Autodesk Inventor part; units mm, degrees
ref_plane "YZ Plane" through (0, 0, 0) normal (1, 0, 0) x (0, 1, 0)
ref_plane "XZ Plane" through (0, 0, 0) normal (0, 1, 0) x (-1, 0, 0)
ref_plane "XY Plane" through (0, 0, 0) normal (0, 0, 1) x (1, 0, 0)
sketch "Sketch1" plane through (0, 0, 0) normal (0, 0, 1) x (1, 0, 0)
  circle A0 centre (3.2816, -5.4552) radius 1.5
  line L0 (4.45, -12.0667) -> (7.65, -10.2192)
  line L1 (7.65, -10.2192) -> (10.85, -12.0667)
  line L2 (10.85, -12.0667) -> (10.85, -15.7617)
  line L3 (10.85, -15.7617) -> (7.65, -17.6093)
  line L4 (7.65, -17.6093) -> (4.45, -15.7617)
  line L5 (4.45, -15.7617) -> (4.45, -12.0667)
  circle A1 centre (3.2816, -22.3733) radius 1.5
  line L6 (15.3, -27.8284) -> (15.3, 0)
  line L7 (0, 0) -> (15.3, 0)
  line L8 (0, -27.8284) -> (0, 0)
  line L9 (0, -27.8284) -> (15.3, -27.8284)
  line L10 (28.3, 5.8858) -> (15.3, 5.8858)
  line L11 (15.3, 5.8858) -> (15.3, -34.1142)
  line L12 (28.3, -34.1142) -> (15.3, -34.1142)
  line L13 (28.3, 5.8858) -> (28.3, -34.1142)
  line L14 (38.8108, -39.1142) -> (38.8108, 10.8858)
  line L15 (38.8108, 10.8858) -> (15.3, 10.8858)
  line L16 (15.3, -2.6142) -> (15.3, 10.8858)
  line L17 (15.3, -2.6142) -> (38.3, -2.6142)
  line L18 (38.3, -12.6142) -> (38.3, -2.6142)
  line L19 (38.3, -12.6142) -> (7.65, -12.6142)
  arc A2 (7.65, -15.6142) -> (7.65, -12.6142) centre (7.65, -14.1142) ccw
  line L20 (7.65, -15.6142) -> (38.3, -15.6142)
  line L21 (38.3, -25.6142) -> (38.3, -15.6142)
  line L22 (38.3, -25.6142) -> (15.3, -25.6142)
  line L23 (15.3, -39.1142) -> (15.3, -25.6142)
  line L24 (38.8108, -39.1142) -> (15.3, -39.1142)
  line L25 (-7.04, -39.1142) -> (14.96, -39.1142)
  line L26 (-7.04, -39.1142) -> (38.8108, -39.1142)
  line L27 (38.8108, -39.1142) -> (38.8108, 10.8858)
  line L28 (38.8108, 10.8858) -> (-7.04, 10.8858)
  line L29 (-7.04, 10.8858) -> (-7.04, -39.1142)
  line L30 (-5.04, -27.8284) -> (13.16, -27.8284)
  line L31 (13.16, 0) -> (-5.04, 0)
  line L32 (-3.04, -35.1142) -> (34.8108, -35.1142)
  line L33 (34.8108, -35.1142) -> (34.8108, 6.8858)
  line L34 (34.8108, 6.8858) -> (-3.04, 6.8858)
  line L35 (-3.04, 6.8858) -> (-3.04, -35.1142)
  line L36 (34.8108, -35.1142) -> (15.3, -35.1142)
  line L37 (15.3, -35.1142) -> (15.3, -39.1142)
  line L38 (15.3, -39.1142) -> (34.8108, -39.1142)
  line L39 (34.8108, -39.1142) -> (34.8108, -35.1142)
  line L40 (15.3, 6.8858) -> (34.8108, 6.8858)
  line L41 (34.8108, 6.8858) -> (34.8108, 10.8858)
  line L42 (34.8108, 10.8858) -> (15.3, 10.8858)
  line L43 (15.3, 10.8858) -> (15.3, 6.8858)
  point P0 (-3.04, 0)
  point P1 (-3.04, -27.8284)
  dimension "d0" = 4
extrude "Extrusion1" add sketch "Sketch1" along normal blind 2 contours L5 L4 L3 L2 L20 L6 L9 L8 L7 L19 L1 L0 | L0 L1 L2 L19 A2 L20 L3 L4 L5 | L19 L6 L20 L2 | L2 L20 A2 L19 | L19 L13 L20 L6 | L6 L17 L13 L19 | L20 L13 L22 L6 | L6 L11 L10 L13 L17 | L19 L33 L20 L13 | L13 L17 L33 L19 | L22 L13 L12 L11 L6 | L20 L33 L22 L13 | L13 L10 L16 L34 L33 L17 | L33 L17 L18 L19 | L19 L18 L17 L33 L41 L15 L14 L24 L39 L22 L21 L20 | L22 L33 L32 L23 L12 L13 | L20 L21 L22 L33 | L8 L30 L35 L31 | L16 L15 L41 L34 | L32 L39 L24 L23
sketch "Sketch2" plane through (0, 0, 2) normal (0, 0, 1) x (1, 0, 0)
  line L0 (15.3, 0) -> (-3.04, 0)
  line L1 (-3.04, 0) -> (-3.04, -27.8284)
  line L2 (-3.04, -27.8284) -> (15.3, -27.8284)
  line L3 (15.3, -27.8284) -> (15.3, -39.1142)
  line L4 (15.3, -39.1142) -> (38.8108, -39.1142)
  line L5 (38.8108, -39.1142) -> (38.8108, 10.8858)
  line L6 (38.8108, 10.8858) -> (15.3, 10.8858)
  line L7 (15.3, 10.8858) -> (15.3, 0)
  circle A0 centre (3.2816, -22.3733) radius 1.5
  circle A1 centre (3.2816, -5.4552) radius 1.5
  line L8 (15.3, -39.1142) -> (38.8108, -39.1142)
  line L9 (38.8108, 10.8858) -> (34.8108, 10.8858)
  line L10 (34.8108, 10.8858) -> (34.8108, -39.1142)
  line L11 (34.8108, -39.1142) -> (38.8108, -39.1142)
  line L12 (38.8108, -39.1142) -> (38.8108, 10.8858)
  point P0 (0, 0)
  dimension "d3" = 4
extrude "Extrusion2" cut sketch "Sketch2" against normal blind 2 contours L6 L5 L4 L10
sketch "Sketch3" plane through (0, 0, 2) normal (0, 0, 1) x (1, 0, 0)
  point P0 (0, 0)
sketch "Sketch4" plane through (0, 0, 2) normal (0, 0, 1) x (1, 0, 0)
  circle A0 centre (16.8, -32.0784) radius 0.75
  circle A1 centre (16.8, 4.25) radius 0.75
  point P0 (0, 0)
extrude "Extrusion3" cut sketch "Sketch4" against normal through all
sketch "Sketch5" plane through (0, 0, 2) normal (0, 0, 1) x (1, 0, 0)
  circle A0 centre (16.8, 4.25) radius 0.75
  circle A1 centre (16.8, -32.0784) radius 0.75
  line L0 (34.8108, -39.1142) -> (34.8108, 10.8858)
  line L1 (34.8108, 10.8858) -> (15.3, 10.8858)
  line L2 (15.3, 10.8858) -> (15.3, 0)
  line L3 (15.3, 0) -> (-3.04, 0)
  line L4 (-3.04, 0) -> (-3.04, -27.8284)
  line L5 (-3.04, -27.8284) -> (15.3, -27.8284)
  line L6 (15.3, -27.8284) -> (15.3, -39.1142)
  line L7 (15.3, -39.1142) -> (34.8108, -39.1142)
  circle A2 centre (3.2816, -22.3733) radius 1.5
  circle A3 centre (3.2816, -5.4552) radius 1.5
  line L8 (22.1108, -36.7142) -> (32.8108, -36.7142)
  line L9 (22.1108, -36.7142) -> (22.1108, -35.1142)
  line L10 (32.8108, -35.1142) -> (22.1108, -35.1142)
  line L11 (32.8108, -36.7142) -> (32.8108, -35.1142)
  line L12 (32.4108, -28.3142) -> (32.4108, -17.6142)
  line L13 (32.4108, -28.3142) -> (30.8108, -28.3142)
  line L14 (30.8108, -17.6142) -> (30.8108, -28.3142)
  line L15 (32.4108, -17.6142) -> (30.8108, -17.6142)
  line L16 (32.4108, -6.3142) -> (32.4108, 4.3858)
  line L17 (32.4108, -6.3142) -> (30.8108, -6.3142)
  line L18 (30.8108, 4.3858) -> (30.8108, -6.3142)
  line L19 (32.4108, 4.3858) -> (30.8108, 4.3858)
  line L20 (32.8108, 8.4858) -> (22.1108, 8.4858)
  line L21 (32.8108, 8.4858) -> (32.8108, 6.8858)
  line L22 (22.1108, 6.8858) -> (32.8108, 6.8858)
  line L23 (22.1108, 8.4858) -> (22.1108, 6.8858)
  point P0 (0, 0)
extrude "Extrusion4" cut sketch "Sketch5" against normal through all contours L9 L10 L11 L8 | L13 L14 L15 L12 | L17 L18 L19 L16 | L21 L22 L23 L20
sketch "Sketch6" plane through (0, 0, 2) normal (0, 0, 1) x (1, 0, 0)
  line L0 (30.8108, -28.3142) -> (30.8108, -17.6142)
  line L1 (30.8108, -17.6142) -> (32.4108, -17.6142)
  line L2 (32.4108, -17.6142) -> (32.4108, -28.3142)
  line L3 (32.4108, -28.3142) -> (30.8108, -28.3142)
  line L4 (30.8108, -6.3142) -> (30.8108, 4.3858)
  line L5 (30.8108, 4.3858) -> (32.4108, 4.3858)
  line L6 (32.4108, 4.3858) -> (32.4108, -6.3142)
  line L7 (32.4108, -6.3142) -> (30.8108, -6.3142)
  line L8 (22.1108, -35.1142) -> (32.8108, -35.1142)
  line L9 (32.8108, -35.1142) -> (32.8108, -36.7142)
  line L10 (32.8108, -36.7142) -> (22.1108, -36.7142)
  line L11 (22.1108, -36.7142) -> (22.1108, -35.1142)
  line L12 (32.8108, 6.8858) -> (22.1108, 6.8858)
  line L13 (22.1108, 6.8858) -> (22.1108, 8.4858)
  line L14 (22.1108, 8.4858) -> (32.8108, 8.4858)
  line L15 (32.8108, 8.4858) -> (32.8108, 6.8858)
  circle A0 centre (16.8, 4.25) radius 0.75
  circle A1 centre (16.8, -32.0784) radius 0.75
  line L16 (34.8108, -39.1142) -> (34.8108, 10.8858)
  line L17 (34.8108, 10.8858) -> (15.3, 10.8858)
  line L18 (15.3, 10.8858) -> (15.3, 0)
  line L19 (15.3, 0) -> (-3.04, 0)
  line L20 (-3.04, 0) -> (-3.04, -27.8284)
  line L21 (-3.04, -27.8284) -> (15.3, -27.8284)
  line L22 (15.3, -27.8284) -> (15.3, -39.1142)
  line L23 (15.3, -39.1142) -> (34.8108, -39.1142)
  circle A2 centre (3.2816, -22.3733) radius 1.5
  circle A3 centre (3.2816, -5.4552) radius 1.5
  line L24 (34.8108, 10.8858) -> (15.3, 10.8858)
  line L25 (15.3, 10.8858) -> (15.3, 0)
  line L26 (34.8108, 10.8858) -> (15.3, 10.8858)
  line L27 (15.3, 10.8858) -> (15.3, 10.0858)
  line L28 (15.3, 10.0858) -> (34.8108, 10.0858)
  line L29 (34.8108, 10.0858) -> (34.8108, 10.8858)
  line L30 (15.3, -27.8284) -> (15.3, -39.1142)
  line L31 (34.8108, 10.8858) -> (34.8108, -39.1142)
  line L32 (15.3, -39.1142) -> (34.8108, -39.1142)
  line L33 (34.8108, -39.1142) -> (34.8108, -38.3142)
  line L34 (34.8108, -38.3142) -> (15.3, -38.3142)
  line L35 (15.3, -38.3142) -> (15.3, -39.1142)
  point P0 (0, 0)
  dimension "d10" = 0.8
  dimension "d11" = 0.8
extrude "Extrusion5" cut sketch "Sketch6" against normal through all contours L23 L22 L34 L16 | L28 L18 L17 L16
sketch "Sketch7" plane through (0, 0, 2) normal (0, 0, 1) x (1, 0, 0)
  line L0 (34.8108, 10.0858) -> (15.3, 10.0858)
  line L1 (15.3, 10.0858) -> (15.3, 0)
  line L2 (15.3, 0) -> (-3.04, 0)
  line L3 (-3.04, 0) -> (-3.04, -27.8284)
  line L4 (-3.04, -27.8284) -> (15.3, -27.8284)
  line L5 (15.3, -27.8284) -> (15.3, -38.3142)
  line L6 (15.3, -38.3142) -> (34.8108, -38.3142)
  line L7 (34.8108, -38.3142) -> (34.8108, 10.0858)
  line L8 (30.8108, -28.3142) -> (30.8108, -17.6142)
  line L9 (30.8108, -17.6142) -> (32.4108, -17.6142)
  line L10 (32.4108, -17.6142) -> (32.4108, -28.3142)
  line L11 (32.4108, -28.3142) -> (30.8108, -28.3142)
  line L12 (30.8108, -6.3142) -> (30.8108, 4.3858)
  line L13 (30.8108, 4.3858) -> (32.4108, 4.3858)
  line L14 (32.4108, 4.3858) -> (32.4108, -6.3142)
  line L15 (32.4108, -6.3142) -> (30.8108, -6.3142)
  line L16 (22.1108, -35.1142) -> (32.8108, -35.1142)
  line L17 (32.8108, -35.1142) -> (32.8108, -36.7142)
  line L18 (32.8108, -36.7142) -> (22.1108, -36.7142)
  line L19 (22.1108, -36.7142) -> (22.1108, -35.1142)
  line L20 (32.8108, 6.8858) -> (22.1108, 6.8858)
  line L21 (22.1108, 6.8858) -> (22.1108, 8.4858)
  line L22 (22.1108, 8.4858) -> (32.8108, 8.4858)
  line L23 (32.8108, 8.4858) -> (32.8108, 6.8858)
  circle A0 centre (16.8, 4.25) radius 0.75
  circle A1 centre (16.8, -32.0784) radius 0.75
  circle A2 centre (3.2816, -22.3733) radius 1.5
  circle A3 centre (3.2816, -5.4552) radius 1.5
  line L24 (38.8108, 10.8858) -> (15.3, 10.8858)
  line L25 (38.8108, -39.1142) -> (15.3, -39.1142)
  line L26 (15.3, 10.0858) -> (34.8108, 10.0858)
  line L27 (15.3, 10.8858) -> (34.8108, 10.8858)
  line L28 (34.8108, 10.8858) -> (34.8108, 10.0858)
  line L29 (34.8108, 10.0858) -> (15.3, 10.0858)
  line L30 (15.3, 10.0858) -> (15.3, 10.8858)
  line L31 (34.8108, -38.3142) -> (15.3, -38.3142)
  line L32 (34.8108, -38.3142) -> (15.3, -38.3142)
  line L33 (15.3, -38.3142) -> (15.3, -39.1142)
  line L34 (15.3, -39.1142) -> (34.8108, -39.1142)
  line L35 (34.8108, -39.1142) -> (34.8108, -38.3142)
  point P0 (0, 0)
extrude "Extrusion6" add sketch "Sketch7" against normal up to surface (2 mm away) contours L0 L30 L24 L28 | L35 L25 L33 L6
sketch "Sketch8" plane through (0, 0, 2) normal (0, 0, 1) x (1, 0, 0)
  line L0 (15.3, 10.8858) -> (15.3, 0)
  line L1 (15.3, 0) -> (-3.04, 0)
  line L2 (-3.04, 0) -> (-3.04, -27.8284)
  line L3 (-3.04, -27.8284) -> (15.3, -27.8284)
  line L4 (15.3, -27.8284) -> (15.3, -39.1142)
  line L5 (15.3, -39.1142) -> (34.8108, -39.1142)
  line L6 (34.8108, -39.1142) -> (34.8108, 10.8858)
  line L7 (34.8108, 10.8858) -> (15.3, 10.8858)
  line L8 (30.8108, -28.3142) -> (30.8108, -17.6142)
  line L9 (30.8108, -17.6142) -> (32.4108, -17.6142)
  line L10 (32.4108, -17.6142) -> (32.4108, -28.3142)
  line L11 (32.4108, -28.3142) -> (30.8108, -28.3142)
  line L12 (30.8108, -6.3142) -> (30.8108, 4.3858)
  line L13 (30.8108, 4.3858) -> (32.4108, 4.3858)
  line L14 (32.4108, 4.3858) -> (32.4108, -6.3142)
  line L15 (32.4108, -6.3142) -> (30.8108, -6.3142)
  line L16 (22.1108, -35.1142) -> (32.8108, -35.1142)
  line L17 (32.8108, -35.1142) -> (32.8108, -36.7142)
  line L18 (32.8108, -36.7142) -> (22.1108, -36.7142)
  line L19 (22.1108, -36.7142) -> (22.1108, -35.1142)
  line L20 (32.8108, 6.8858) -> (22.1108, 6.8858)
  line L21 (22.1108, 6.8858) -> (22.1108, 8.4858)
  line L22 (22.1108, 8.4858) -> (32.8108, 8.4858)
  line L23 (32.8108, 8.4858) -> (32.8108, 6.8858)
  circle A0 centre (16.8, 4.25) radius 0.75
  circle A1 centre (16.8, -32.0784) radius 0.75
  circle A2 centre (3.2816, -22.3733) radius 1.5
  circle A3 centre (3.2816, -5.4552) radius 1.5
  line L24 (28.5108, 8.4858) -> (17.8108, 8.4858)
  line L25 (28.5108, 8.4858) -> (28.5108, 6.8858)
  line L26 (17.8108, 6.8858) -> (28.5108, 6.8858)
  line L27 (17.8108, 8.4858) -> (17.8108, 6.8858)
  point P0 (0, 0)
extrude "Extrusion7" cut sketch "Sketch8" against normal blind 10 contours L26 L27 L24 L21
sketch "Sketch9" plane through (0, 0, 2) normal (0, 0, 1) x (1, 0, 0)
  circle A0 centre (3.2816, -5.4552) radius 1.5
  circle A1 centre (3.2816, -22.3733) radius 1.5
  circle A2 centre (16.8, -32.0784) radius 0.75
  circle A3 centre (16.8, 4.25) radius 0.75
  line L0 (32.8108, 6.8858) -> (17.8108, 6.8858)
  line L1 (17.8108, 6.8858) -> (17.8108, 8.4858)
  line L2 (17.8108, 8.4858) -> (32.8108, 8.4858)
  line L3 (32.8108, 8.4858) -> (32.8108, 6.8858)
  line L4 (22.1108, -35.1142) -> (32.8108, -35.1142)
  line L5 (32.8108, -35.1142) -> (32.8108, -36.7142)
  line L6 (32.8108, -36.7142) -> (22.1108, -36.7142)
  line L7 (22.1108, -36.7142) -> (22.1108, -35.1142)
  line L8 (30.8108, -6.3142) -> (30.8108, 4.3858)
  line L9 (30.8108, 4.3858) -> (32.4108, 4.3858)
  line L10 (32.4108, 4.3858) -> (32.4108, -6.3142)
  line L11 (32.4108, -6.3142) -> (30.8108, -6.3142)
  line L12 (30.8108, -28.3142) -> (30.8108, -17.6142)
  line L13 (30.8108, -17.6142) -> (32.4108, -17.6142)
  line L14 (32.4108, -17.6142) -> (32.4108, -28.3142)
  line L15 (32.4108, -28.3142) -> (30.8108, -28.3142)
  line L16 (15.3, 10.8858) -> (15.3, 0)
  line L17 (15.3, 0) -> (-3.04, 0)
  line L18 (-3.04, 0) -> (-3.04, -27.8284)
  line L19 (-3.04, -27.8284) -> (15.3, -27.8284)
  line L20 (15.3, -27.8284) -> (15.3, -39.1142)
  line L21 (15.3, -39.1142) -> (34.8108, -39.1142)
  line L22 (34.8108, -39.1142) -> (34.8108, 10.8858)
  line L23 (34.8108, 10.8858) -> (15.3, 10.8858)
  line L24 (28.5108, 8.4858) -> (28.5108, 6.8858)
  point P0 (0, 0)
extrude "Extrusion8" add sketch "Sketch9" against normal up to surface (2 mm away) contours L0 L24 L2 L3
properties part number "pcbek"
Geometry check sheet. Reference: the model listing, model coordinates, mm. A direction names the side the tool comes from. Give positions to 0.01 mm unless a question says otherwise; leave off trailing zeros. Order: outer loops, then holes, each group sorted by start corner. A loop starts at its lowest first (then second) coordinate and runs counter-clockwise, first axis right, second up.
1) Tool access check on faces 4 (the flat face through (34.811, -14, 1)), 5 (the flat face through (15.3, 6, 1)), 6 (the flat face through (30.811, -1, 1)). Record the directions out of +Z, -Z, +X, -X, +Y, -Y that give a thin tool (end or side, any length) a straight path to the whole face; none if there is none.
Results are:
face 4: +Z, -Z, +X, +Y, -Y
face 5: +Z, -Z, -X, +Y
face 6: +Z, -Z
2) Cross-section at B-B (y = -19). Record the boundary of the cut face in (x, z), then the cut area to 3 significant figures.
Results are:
outline: (-3.04, 0) - (30.81, 0) - (30.81, 2) - (-3.04, 2) - close; (32.41, 0) - (34.81, 0) - (34.81, 2) - (32.41, 2) - close
area: 72.5 mm2
3) Draft check along Y on faces 1 (the flat face through (6, -27.828, 1)), 2 (the flat face through (15.3, -33, 1)), 3 (the flat face through (17.811, 8, 1)). Enter one of: released by +Y, released by -Y, zero draft, split by the parting line, or undercut.
Results are:
face 1: released by -Y
face 2: zero draft
face 3: undercut
4) Gauge pin test, flat ends, axial feed: pin 1 (1 mm diameter, centred on x = 9, z = 0.5, fed in from +Y); pin 2 (1 mm diameter, centred on y = 8, z = 1.5, fed in from -X). Record the tip position at first contact, or that the pin passes through.
Results are:
pin 1: stops at y = 0
pin 2: stops at x = 15.3
5) Cross-section at A-A (x = 20). Record the boundary of the cut face in (y, z).
Results are:
outline: (-39.11, 0) - (6.89, 0) - (6.89, 2) - (-39.11, 2) - close; (8.49, 0) - (10.89, 0) - (10.89, 2) - (8.49, 2) - close
6) Material ranges on probe 1 along Y at (x, z) = (16.8, 1.2); probe 2 along Y at (x, z) = (17, 0.4); probe 3 along X at (y, z) = (7.5, 0.7), recorded low to high.
Results are:
probe 1: y = -39.11 to -32.83, -31.33 to 3.5, 5 to 10.89
probe 2: y = -39.11 to -32.8, -31.36 to 3.53, 4.97 to 10.89
probe 3: x = 15.3 to 17.81, 28.51 to 34.81
7) Cross-section at D-D (z = 0.7). Give the number of separate pieces and of enclosed holes in the cut face, then the cut area to 3 significant figures.
Results are:
separate pieces: 1
enclosed holes: 8
area: 1,400 mm2
8) Cross-section at C-C (x = 24). Record the boundary of the cut face in (y, z).
Results are:
outline: (-39.11, 0) - (-36.71, 0) - (-36.71, 2) - (-39.11, 2) - close; (-35.11, 0) - (6.89, 0) - (6.89, 2) - (-35.11, 2) - close; (8.49, 0) - (10.89, 0) - (10.89, 2) - (8.49, 2) - close
